```python
from build123d import *

# Parameters (mm, degrees)
BOSS_EXTRUDE1_DEPTH = 38.1
SKETCH2_R           = 4.2164
CUT_EXTRUDE1_DEPTH  = 38.1
SKETCH3_R           = 4.2164
BOSS_EXTRUDE2_DEPTH = 6.096
BOSS_EXTRUDE3_DEPTH = 1.7145


with BuildPart() as part:
    # Sketch1 → Boss-Extrude1 (new body)
    with BuildSketch(Plane.XY):
        with BuildLine():
            Line((-19.05, -12.7), (-19.05, 12.7))
            Line((-19.05, 12.7), (19.05, 12.7))
            Line((19.05, 12.7), (19.05, -12.7))
            ThreePointArc((19.05, -12.7), (0, -31.75), (-19.05, -12.7))
        make_face()
    extrude(amount=BOSS_EXTRUDE1_DEPTH)

    # Sketch2 → Cut-Extrude1 (cut)
    with BuildSketch(Plane(origin=(0, 0, 0), x_dir=(-1, 0, 0), z_dir=(0, 0, -1))):
        with Locations((0, -12.7)):
            Circle(SKETCH2_R)
    extrude(amount=-CUT_EXTRUDE1_DEPTH, mode=Mode.SUBTRACT)

    # Sketch3 → Boss-Extrude2 (add)
    with BuildSketch(Plane(origin=(0, 12.7, 0), x_dir=(1, 0, 0), z_dir=(0, 1, 0))):
        with Locations(Location((0, -19.05, 0), (0, 0, 90))):
            Circle(SKETCH3_R)
    extrude(amount=BOSS_EXTRUDE2_DEPTH)

    # Sketch4 → Boss-Extrude3 (add)
    with BuildSketch(Plane(origin=(0, 18.796, 0), x_dir=(1, 0, 0), z_dir=(0, 1, 0))):
        with BuildLine():
            Line((-4.2164, -27.559), (-4.2164, -10.541))
            ThreePointArc((-4.2164, -10.541), (0, -6.3246), (4.2164, -10.541))
            Line((4.2164, -10.541), (4.2164, -27.559))
            ThreePointArc((4.2164, -27.559), (0, -31.7754), (-4.2164, -27.559))
        make_face()
    extrude(amount=-BOSS_EXTRUDE3_DEPTH)


solid = part.part
```
Geometry: final body of the model. Coordinates: model frame, mm. A direction names the side the tool comes from. Round coordinates to 2 decimals unless told otherwise and drop trailing zeros. Order: outer loops, then holes, each group sorted by start corner. A loop starts at its lowest first (then second) coordinate and runs counter-clockwise, first axis right, second up. Notation, with made-up numbers: (8.5, 57.25) -> (57.5, 57.25) arc R25 cw to (57.5, 83.25) -> close; hole circle Ø2 at (-1, 34). An arc over 180 degrees is marked (long way). Use CSV: the item, a comma, the result in double quotes. Start each with the question number.
1) Section C-C (z = 21.5). Return the cut outline in (x, y), and give its area (3 significant figures).
2) First-contact query: pin 1 Ø2 at (y, z) = (-24.5, 13.5) entering from +X; pin 2 Ø5 at (x, y) = (-10.5, 12) entering from -Z; pin 3 Ø1 at (y, z) = (-18.5, 11) entering from -X; pin 4 Ø0.9 at (y, z) = (18.5, 21) entering from +X. Flat tips, straight axial feed; report the tip coordinate or a pass-through.
3) Draft query along Y for faces 6 (the face through (0.419, -31.745, 18.783)), 7 (the face through (4.216, 18, 19)), 8 (the face through (0.55, -8.52, 18.78)). Return one class per face: +Y half, -Y half, draft (parallel to the pull), parting line (faces both ways), or undercut.
4) Section B-B (z = 31). Return the cut outline in (x, y), and give its area (3 significant figures).
5) Section D-D (y = -21). Return the cut outline in (x, z), and give its area (3 significant figures).
6) Set-up query: faces 1 (the face through (-4.216, 18, 19)), 2 (the face through (-2.8, 14.9, 22.2)), 3 (the face through (-0.093, 17.951, 6.326)), 4 (the face through (0.093, 17.951, 31.774)), 5 (the face through (0, -4, 38.1)). Return all of +Z, -Z, +X, -X, +Y, -Y with unobstructed straight access to the full face (end or side cutting, diameter ignored); none if empty.
7) Section A-A (x = 0). Return the cut outline in (y, z), and give its area (3 significant figures).
8) Material intervals for line 1 along Y through (x, z) = (0, 10); line 2 along Y through (x, z) = (0, 20); line 3 along X through (y, z) = (-12, 11), sorted ascending. Write a range as from..to.
Returned:
1,outline,"(-19.05, -12.7) arc R19.05 ccw to (19.05, -12.7) -> (19.05, 12.7) -> (3.43, 12.7) -> (3.43, 17.08) -> (4.22, 17.08) -> (4.22, 18.8) -> (-4.22, 18.8) -> (-4.22, 17.08) -> (-3.43, 17.08) -> (-3.43, 12.7) -> (-19.05, 12.7) -> close; hole circle Ø8.43 at (0, -12.7)"
1,area,"1,530 mm²"
2,pin 1,"stops at x = 15.69"
2,pin 2,"stops at z = 0"
2,pin 3,"stops at x = -18.3"
2,pin 4,"stops at x = 4.22"
3,face 6,"-Y half"
3,face 7,"draft"
3,face 8,"undercut"
4,outline,"(-19.05, -12.7) arc R19.05 ccw to (19.05, -12.7) -> (19.05, 12.7) -> (-19.05, 12.7) -> close; (-2.44, 17.08) -> (2.44, 17.08) -> (2.44, 18.8) -> (-2.44, 18.8) -> close; hole circle Ø8.43 at (0, -12.7)"
4,area,"1,490 mm²"
5,outline,"(-17.15, 0) -> (17.15, 0) -> (17.15, 38.1) -> (-17.15, 38.1) -> close"
5,area,"1,310 mm²"
6,face 1,"+Z, -Z, -X, +Y"
6,face 2,"none"
6,face 3,"-Z, +Y"
6,face 4,"+Z, +Y"
6,face 5,"+Z, +X, -X, +Y, -Y"
7,outline,"(-31.75, 0) -> (-16.92, 0) -> (-16.92, 38.1) -> (-31.75, 38.1) -> close; (-8.48, 0) -> (12.7, 0) -> (12.7, 14.83) -> (17.08, 14.83) -> (17.08, 6.32) -> (18.8, 6.32) -> (18.8, 31.78) -> (17.08, 31.78) -> (17.08, 23.27) -> (12.7, 23.27) -> (12.7, 38.1) -> (-8.48, 38.1) -> close"
7,area,"1,450 mm²"
8,line 1,"y = -31.75..-16.92, -8.48..12.7, 17.08..18.8"
8,line 2,"y = -31.75..-16.92, -8.48..18.8"
8,line 3,"x = -19.05..-4.16, 4.16..19.05"
